```python
from build123d import *

# Parameters (mm, degrees)
SKETCH1_R           = 2.4892
SKETCH1_W           = 25.4
SKETCH1_H           = 76.2
BOSS_EXTRUDE1_DEPTH = 6.35
FILLET1_R           = 6.35


with BuildPart() as part:
    # Sketch1 → Boss-Extrude1 (new body)
    # profile 1 of 3: a face of its own
    with BuildSketch(Plane(origin=(0, 0, 0), x_dir=(1, 0, 0), z_dir=(0, 1, 0))):
        with BuildLine():
            Line((-38.1, 76.2), (0, 76.2))
            Line((0, 76.2), (0, 86.4108))
            ThreePointArc((0, 86.4108), (-2.4892, 88.9), (0, 91.3892))
            Line((0, 91.3892), (0, 101.6))
            Line((0, 101.6), (-38.1, 101.6))
            Line((-38.1, 101.6), (-38.1, 76.2))
        make_face()
        with Locations(Location((-25.4, 88.9, 0), (0, 0, 270))):
            Circle(SKETCH1_R, mode=Mode.SUBTRACT)
        with Locations(Location((-12.7, 88.9, 0), (0, 0, 270))):
            Circle(SKETCH1_R, mode=Mode.SUBTRACT)
    # profile 2 of 3: a face of its own
    with BuildSketch(Plane(origin=(0, 0, 0), x_dir=(1, 0, 0), z_dir=(0, 1, 0))):
        with BuildLine():
            Line((0, 86.4108), (0, 76.2))
            Line((0, 76.2), (25.4, 76.2))
            Line((25.4, 76.2), (25.4, 101.6))
            Line((25.4, 101.6), (0, 101.6))
            Line((0, 101.6), (0, 91.3892))
            ThreePointArc((0, 91.3892), (1.7601302, 90.6601302), (2.4892, 88.9))
            ThreePointArc((2.4892, 88.9), (1.7601302, 87.1398698), (0, 86.4108))
        make_face()
        with Locations(Location((12.7, 88.9, 0), (0, 0, 270))):
            Circle(SKETCH1_R, mode=Mode.SUBTRACT)
    # profile 3 of 3: a face of its own
    with BuildSketch(Plane(origin=(0, 0, 0), x_dir=(1, 0, 0), z_dir=(0, 1, 0))):
        with Locations((12.7, 38.1)):
            Rectangle(SKETCH1_W, SKETCH1_H)
        with Locations(Location((12.7, 12.7, 0), (0, 0, 270))):
            Circle(SKETCH1_R, mode=Mode.SUBTRACT)
        with Locations(Location((12.7, 25.4, 0), (0, 0, 270))):
            Circle(SKETCH1_R, mode=Mode.SUBTRACT)
        with Locations(Location((12.7, 38.1, 0), (0, 0, 270))):
            Circle(SKETCH1_R, mode=Mode.SUBTRACT)
        with Locations(Location((12.7, 50.8, 0), (0, 0, 270))):
            Circle(SKETCH1_R, mode=Mode.SUBTRACT)
        with Locations(Location((12.7, 63.5, 0), (0, 0, 270))):
            Circle(SKETCH1_R, mode=Mode.SUBTRACT)
    extrude(amount=BOSS_EXTRUDE1_DEPTH)

    # Fillet1
    fillet1_edges = [part.edges().sort_by_distance(p)[0] for p in [
        (25.4, 3.175, 0),
        (0, 3.175, 0),
        (0, 3.175, -76.2),
        (-38.1, 3.175, -76.2),
        (-38.1, 3.175, -101.6),
        (25.4, 3.175, -101.6),
    ]]
    fillet(fillet1_edges, radius=FILLET1_R)


solid = part.part
```
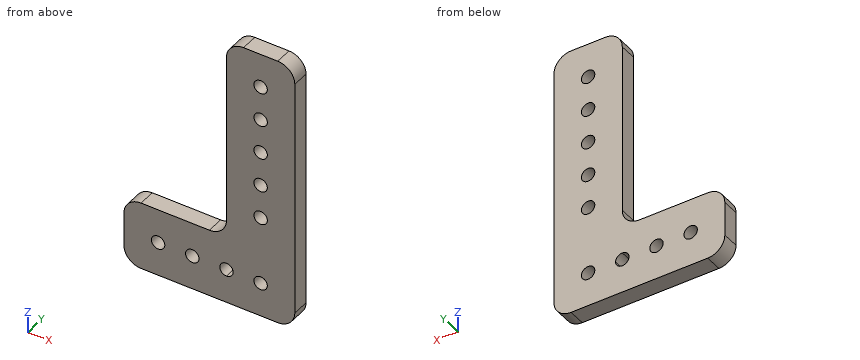
The listing builds one solid part. Answer for the finished solid, in the listing's coordinates (mm). Round coordinates to 2 decimals unless told otherwise and drop trailing zeros. Loops run counter-clockwise (first coordinate to the right, second up) from the corner with the lowest first, then second, coordinate; pieces in that order, holes last.
Q1. Section C-C, the plane y = 4 is taken. Count the separate pieces of the cut face and the enclosed holes in it, then the cut area to 3 significant figures.
Q2. Given pin 1 Ø6.5 at (x, z) = (12.7, -50.8) entering from -Y; pin 2 Ø4 at (x, z) = (12.7, -25.4) entering from +Y; pin 3 Ø2 at (x, y) = (-29, 2) entering from +Z, each flat-ended and moving along its own axis, determine where each tip first touches the part or whether it passes through.
Q3. Find the intervals of material crossed by line 1 (X direction, y = 2.25, z = -88.9); line 2 (X direction, y = 3, z = -50.8); line 3 (Z direction, x = -15.5, y = 5.25), in increasing order.
Q4. Section B-B, the plane z = -38.1 is taken. Determine the outline of the cut face in (x, y).
Q5. Section D-D, the plane x = -12.7 is taken. Determine the outline of the cut face in (y, z).
Q6. Section A-A, the plane x = 12.7 is taken. Determine the outline of the cut face in (y, z), then the cut area to 3 significant figures.
Completed:
1. separate pieces: 1
1. enclosed holes: 9
1. area: 3,340 mm2
2. pin 1: stops at y = 0
2. pin 2: passes through
2. pin 3: stops at z = -76.2
3. line 1: x = -38.1 to -27.89, -22.91 to -15.19, -10.21 to -2.49, 2.49 to 10.21, 15.19 to 25.4
3. line 2: x = 0 to 10.21, 15.19 to 25.4
3. line 3: z = -101.6 to -76.2
4. outline: (0, 0) - (10.21, 0) - (10.21, 6.35) - (0, 6.35) - close; (15.19, 0) - (25.4, 0) - (25.4, 6.35) - (15.19, 6.35) - close
5. outline: (0, -101.6) - (6.35, -101.6) - (6.35, -91.39) - (0, -91.39) - close; (0, -86.41) - (6.35, -86.41) - (6.35, -76.2) - (0, -76.2) - close
6. outline: (0, -101.6) - (6.35, -101.6) - (6.35, -91.39) - (0, -91.39) - close; (0, -86.41) - (6.35, -86.41) - (6.35, -65.99) - (0, -65.99) - close; (0, -61.01) - (6.35, -61.01) - (6.35, -53.29) - (0, -53.29) - close; (0, -48.31) - (6.35, -48.31) - (6.35, -40.59) - (0, -40.59) - close; (0, -35.61) - (6.35, -35.61) - (6.35, -27.89) - (0, -27.89) - close; (0, -22.91) - (6.35, -22.91) - (6.35, -15.19) - (0, -15.19) - close; (0, -10.21) - (6.35, -10.21) - (6.35, 0) - (0, 0) - close
6. area: 455 mm2
